CAD build for the part. Positions are in the model's coordinates, mm. A direction names the side the tool comes from. Round coordinates to 2 decimals unless told otherwise and drop trailing zeros. Order: outer loops, then holes, each group sorted by start corner. A loop starts at its lowest first (then second) coordinate and runs counter-clockwise, first axis right, second up. Notation, with made-up numbers: M 32,-11 L 39,-11 A21 ccw 39,10 Z; hole C 9.25,20 d1. An arc over 180 degrees is marked long. Put each result on its own line as item: value.
```python
from build123d import *

# Parameters (mm, degrees)
SLOT_CUT_EXTRUDE1_DEPTH      = 9.685758617
SLOT_CUT_EXTRUDE1_DEPTH_BACK = 9.685758617
SKETCH2_W                    = 0.6
SKETCH2_H                    = 0.8


with BuildPart() as part:
    # Sketch1 → base-Revolve (revolve)
    with BuildSketch(Plane.XY, mode=Mode.PRIVATE) as base_revolve_sk:
        with BuildLine():
            Line((0, 0), (0, 2.221903197))
            ThreePointArc((0, 2.221903197), (0.098154896, 2.37597552), (0.279273894, 2.352130752))
            Line((0.279273894, 2.352130752), (1.532709575, 1.300373334))
            ThreePointArc((1.532709575, 1.300373334), (1.713170055, 1.196184428), (1.918382141, 1.16))
            Line((1.918382141, 1.16), (2.51, 1.16))
            Line((2.51, 1.16), (2.8, 1.45))
            Line((2.8, 1.45), (8, 1.45))
            Line((8, 1.45), (8, 0))
            Line((8, 0), (0, 0))
        make_face()
    revolve(base_revolve_sk.sketch.rotate(Axis((0, 0, 0), (1, 0, 0)), 90), axis=Axis((0, 0, 0), (1, 0, 0)))

    # Sketch2 → slot_Cut-Extrude1 (cut, two sides: drawn at the far end of the back side and taken through both)
    with BuildSketch(Plane.XY.offset(-SLOT_CUT_EXTRUDE1_DEPTH_BACK)):
        with Locations((0.3, 0)):
            Rectangle(SKETCH2_W, SKETCH2_H)
    extrude(amount=SLOT_CUT_EXTRUDE1_DEPTH + SLOT_CUT_EXTRUDE1_DEPTH_BACK, mode=Mode.SUBTRACT)

    # Sketch8 → point_Cut-Revolve1 (revolve, cut)
    with BuildSketch(Plane.XY, mode=Mode.PRIVATE) as point_cut_revolve1_sk:
        Polygon((8, 0), (8.508, 0), (8.508, 1.958), (7.229237391, 1.958), (7.229237391, 1.45), (8, 1.005), align=None)
    revolve(point_cut_revolve1_sk.sketch.rotate(Axis((0, 0, 0), (1, 0, 0)), 90), axis=Axis((0, 0, 0), (1, 0, 0)), mode=Mode.SUBTRACT)


solid = part.part
```
Item 1: Tool access for faces 1 (the cylindrical face through (2.218, 1.132, -0.251)), 2 (the flat face through (0, -1, 0)): list every direction of +Z, -Z, +X, -X, +Y, -Y with a clear straight run to the whole face (end or side of a thin tool).
Answers below:
face 1: none
face 2: +Z, -Z, -X, +Y, -Y
Item 2: Band-saw the part on B-B on y = 0. Give the cut face in (x, z) (3 decimals), and give its area (3 significant figures).
Answers below:
outline: M 0.6,-2.083 L 1.533,-1.3 A0.6 cw 1.918,-1.16 L 2.51,-1.16 L 2.8,-1.45 L 7.229,-1.45 L 8,-1.005 L 8,1.005 L 7.229,1.45 L 2.8,1.45 L 2.51,1.16 L 1.918,1.16 A0.6 cw 1.533,1.3 L 0.6,2.083 Z
area: 21.0 mm²
Item 3: Mould opens along Y. For faces 3 (the cylindrical face through (5.05, -0.06, -1.45)), 4 (the flat face through (0, 1, 0)), 5 (the flat face through (0.6, 0, 0)) say: pulls with the +Y half, pulls with the -Y half, needs draft (parallel to the pull), parting line crosses it, or undercut.
Answers below:
face 3: parting line crosses it
face 4: needs draft
face 5: undercut
Item 4: Band-saw the part on C-C on x = 6.75. Give the cut face in (y, z), and give its area (3 significant figures).
Answers below:
outline: C 0,0 d2.9
area: 6.61 mm²
Item 5: Band-saw the part on A-A on z = 0. Give the cut face in (x, y) (3 decimals).
Answers below:
outline: M 0,-2.222 A0.17 ccw 0.279,-2.352 L 1.533,-1.3 A0.6 cw 1.918,-1.16 L 2.51,-1.16 L 2.8,-1.45 L 7.229,-1.45 L 8,-1.005 L 8,1.005 L 7.229,1.45 L 2.8,1.45 L 2.51,1.16 L 1.918,1.16 A0.6 cw 1.533,1.3 L 0.279,2.352 A0.17 ccw 0,2.222 L 0,0.4 L 0.6,0.4 L 0.6,-0.4 L 0,-0.4 Z
Item 6: Probe line 1 along Y through (x, z) = (0.5, 0.4); line 2 along X through (y, z) = (-0.3, -1.35); line 3 along X through (y, z) = (-1, -0.75). List the from-to ranges inside material, lowest first. Write a range as [from, to].
Answers below:
line 1: [-2.13, -0.4], [0.4, 2.13]
line 2: [0.6, 1.43], [2.73, 7.35]
line 3: [0, 1.6], [2.6, 7.58]
Item 7: Pin check, flat tips, straight feed: P1, Ø0.6, axis at y = 0, z = 0.5, coming from the -X side; P2, Ø0.5, axis at x = 0, z = -0.5, coming from the +Y side; P3, Ø2, axis at x = 5, z = 1, coming from the +Y side. Stop position of each tip, or through.
Answers below:
P1: x = 0.6
P2: y = 2.37
P3: y = 1.45
